For this review, take the finished solid that the model builds, in its own axes (mm). Face numbers are marked on the shaded views. A direction names the side the tool comes from. Give positions to 0.01 mm unless a question says otherwise; leave off trailing zeros. Order: outer loops, then holes, each group sorted by start corner. A loop starts at its lowest first (then second) coordinate and runs counter-clockwise, first axis right, second up. Notation, with made-up numbers: (23, 75.5) -> (29, 75.5) arc R11 ccw to (29, 92.5) -> close; hole circle Ø2 at (-31.5, -17.5). An arc over 180 degrees is marked (long way). One line per item, written item: value. Start each with the question number.
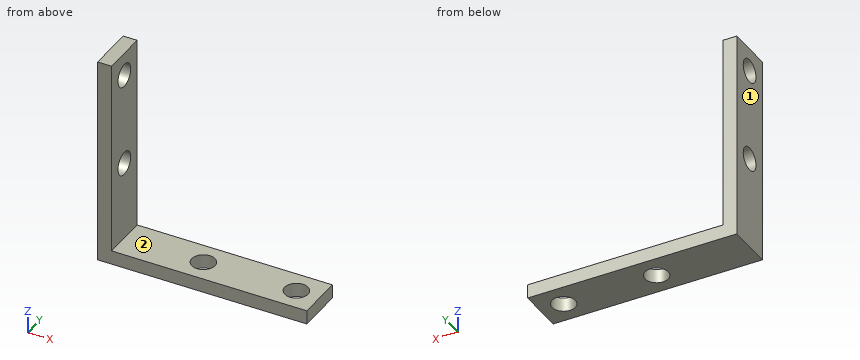
from build123d import *

# Parameters (mm, degrees)
SKETCH1_W           = 45
SKETCH1_H           = 10
SKETCH1_R           = 2.5
BOSS_EXTRUDE1_DEPTH = 3
SKETCH2_W           = 3
SKETCH2_H           = 10
BOSS_EXTRUDE2_DEPTH = 42
SKETCH3_R           = 2.5
CUT_EXTRUDE1_DEPTH  = 3


with BuildPart() as part:
    # Sketch1 → Boss-Extrude1 (new body)
    with BuildSketch(Plane.XY):
        with Locations((22.5, 5)):
            Rectangle(SKETCH1_W, SKETCH1_H)
        with Locations((20, 5)):
            Circle(SKETCH1_R, mode=Mode.SUBTRACT)
        with Locations((40, 5)):
            Circle(SKETCH1_R, mode=Mode.SUBTRACT)
    extrude(amount=BOSS_EXTRUDE1_DEPTH)

    # Sketch2 → Boss-Extrude2 (add)
    with BuildSketch(Plane.XY.offset(3)):
        with Locations((1.5, 5)):
            Rectangle(SKETCH2_W, SKETCH2_H)
    extrude(amount=BOSS_EXTRUDE2_DEPTH)

    # Sketch3 → Cut-Extrude1 (cut)
    with BuildSketch(Plane(origin=(3, 0, 0), x_dir=(0, 0, -1), z_dir=(1, 0, 0))):
        with Locations(Location((-20, 5, 0), (0, 0, 90))):
            Circle(SKETCH3_R)
        with Locations(Location((-40, 5, 0), (0, 0, 90))):
            Circle(SKETCH3_R)
    extrude(amount=-CUT_EXTRUDE1_DEPTH, mode=Mode.SUBTRACT)


solid = part.part
Q1. For the marked faces 1 and 2, list the 3-axis set-ups (+Z, -Z, +X, -X, +Y, -Y) from which the entire face can be reached by the end or side of a thin tool; tool diameter is ignored.
Q2. Take a section at A-A (z = 40). State the section outline as (x, y) points.
Q3. Take a section at C-C (y = 3.25). State the section outline as (x, z) points.
Q4. For line 1 along Z through (x, y) = (2.3, 5); line 2 along Y through (x, z) = (40, 2.2); line 3 along Z through (x, y) = (21.5, 1.25), list the stretches that pass through material, from the lowest coordinate up.
Q5. Take a section at B-B (x = 40). State the section outline as (y, z) points, and give its area (3 significant figures).
Q6. For pin 1 Ø3 at (x, y) = (40, 5) entering from +Z; pin 2 Ø3 at (y, z) = (7, 33) entering from -X; pin 3 Ø6 at (x, y) = (20, 5) entering from +Z; pin 4 Ø5 at (y, z) = (7, 26.5) entering from +X, all flat-tipped, find the tip position at first contact; note any pin that passes through.
Q7. Take a section at D-D (y = 8.5). State the section outline as (x, z) points, and give its area (3 significant figures).
Answers below:
1. face 1: +Z, -Z, -X, +Y, -Y
1. face 2: +Z, +X, +Y, -Y
2. outline: (0, 0) -> (3, 0) -> (3, 2.5) -> (0, 2.5) -> close; (0, 7.5) -> (3, 7.5) -> (3, 10) -> (0, 10) -> close
3. outline: (0, 0) -> (18.21, 0) -> (18.21, 3) -> (3, 3) -> (3, 18.21) -> (0, 18.21) -> close; (0, 21.79) -> (3, 21.79) -> (3, 38.21) -> (0, 38.21) -> close; (0, 41.79) -> (3, 41.79) -> (3, 45) -> (0, 45) -> close; (21.79, 0) -> (38.21, 0) -> (38.21, 3) -> (21.79, 3) -> close; (41.79, 0) -> (45, 0) -> (45, 3) -> (41.79, 3) -> close
4. line 1: z = 0 to 17.5, 22.5 to 37.5, 42.5 to 45
4. line 2: y = 0 to 2.5, 7.5 to 10
4. line 3: z = 0 to 3
5. outline: (0, 0) -> (2.5, 0) -> (2.5, 3) -> (0, 3) -> close; (7.5, 0) -> (10, 0) -> (10, 3) -> (7.5, 3) -> close
5. area: 15.0 mm²
6. pin 1: passes through
6. pin 2: stops at x = 0
6. pin 3: stops at z = 3
6. pin 4: stops at x = 3
7. outline: (0, 0) -> (45, 0) -> (45, 3) -> (3, 3) -> (3, 45) -> (0, 45) -> close
7. area: 261 mm²
